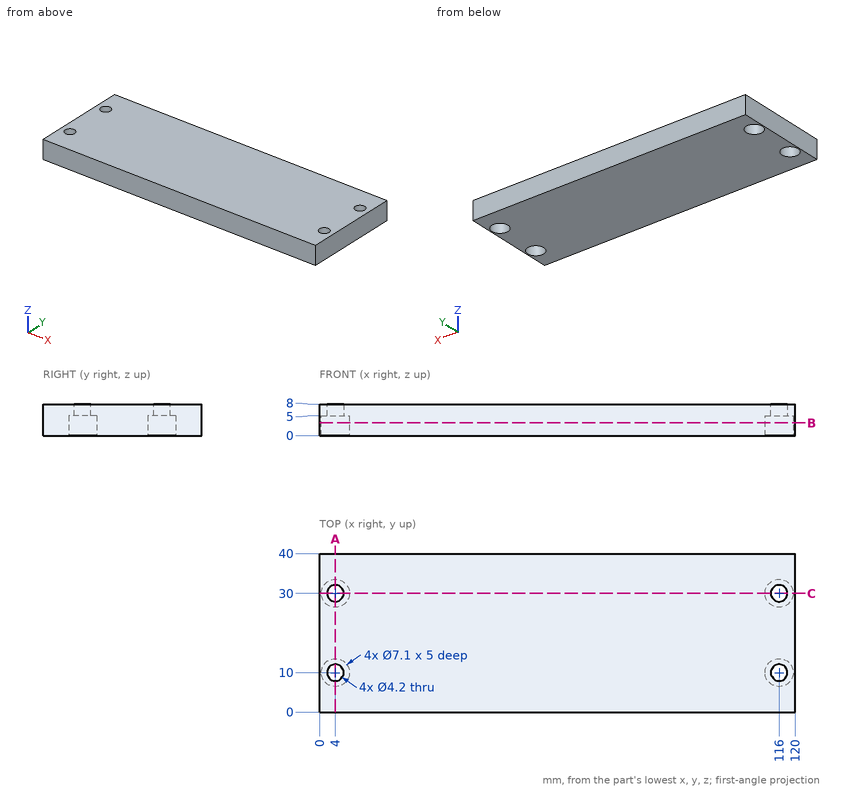
Answer from the drawing. Dimensions are ordinates in mm from the lowest x, y and z of the part. Give positions to 0.01 mm unless a question says otherwise; leave off trailing zeros. Order: outer loops, then holes, each group sorted by start corner. A loop starts at its lowest first (then second) coordinate and runs counter-clockwise, first axis right, second up. Notation, with made-up numbers: (7, 9) -> (58, 9) arc R19 ccw to (58, 14) -> close; hole circle Ø10 at (2.5, 86). An arc over 180 degrees is marked (long way). Answer as a JSON object with one key per item and string values. Group by question number.
1. Section C-C on y = 30 is taken. Determine the outline of the cut face in (x, z), plus the area to 3 significant figures.
2. Consider line 1 along X through (y, z) = (28.5, 7.5); line 2 along X through (y, z) = (13, 3.75). Determine where each line is inside the solid, lowest interval first. Write a range as [from, to].
3. A flat-ended cylindrical pin translates along its axis: pin 1 Ø5.5 at (x, y) = (116, 30) entering from -Z. Find the tip coordinate at first contact, or state that the pin passes through.
4. Section B-B on z = 3.25 is taken. Determine the outline of the cut face in (x, y).
5. Section A-A on x = 4 is taken. Determine the outline of the cut face in (y, z), plus the area to 3 significant figures.
Result sheet:
{
 "1": {"outline": "(0, 0) -> (0.45, 0) -> (0.45, 5) -> (1.9, 5) -> (1.9, 8) -> (0, 8) -> close; (6.1, 5) -> (7.55, 5) -> (7.55, 0) -> (112.45, 0) -> (112.45, 5) -> (113.9, 5) -> (113.9, 8) -> (6.1, 8) -> close; (118.1, 5) -> (119.55, 5) -> (119.55, 0) -> (120, 0) -> (120, 8) -> (118.1, 8) -> close", "area": "864 mm^2"},
 "2": {"line 1": "x = [0, 2.53], [5.47, 114.53], [117.47, 120]", "line 2": "x = [0, 2.1], [5.9, 114.1], [117.9, 120]"},
 "3": {"pin 1": "stops at z = 5"},
 "4": {"outline": "(0, 0) -> (120, 0) -> (120, 40) -> (0, 40) -> close; hole circle Ø7.1 at (4, 10); hole circle Ø7.1 at (4, 30); hole circle Ø7.1 at (116, 10); hole circle Ø7.1 at (116, 30)"},
 "5": {"outline": "(0, 0) -> (6.45, 0) -> (6.45, 5) -> (7.9, 5) -> (7.9, 8) -> (0, 8) -> close; (12.1, 5) -> (13.55, 5) -> (13.55, 0) -> (26.45, 0) -> (26.45, 5) -> (27.9, 5) -> (27.9, 8) -> (12.1, 8) -> close; (32.1, 5) -> (33.55, 5) -> (33.55, 0) -> (40, 0) -> (40, 8) -> (32.1, 8) -> close", "area": "224 mm^2"}
}
